Design review of the part built by this model. Coordinates are the model's own, in mm. A direction names the side the tool comes from. Coordinates: 2 decimals unless noted, no trailing zeros. Write each loop counter-clockwise with the first axis right and the second up, starting at its lowest first coordinate (ties: lowest second). Pieces come first, ordered by that corner, then holes. Notation, with made-up numbers: (-39.5, 15.25) - (-33.5, 15.25) arc R10 cw to (-33.5, 19.25) - close; hole circle Ø7 at (50.5, 17.5). An arc over 180 degrees is marked (long way). Answer as a JSON object with one key per item and string values.
```python
from build123d import *

# Parameters (mm, degrees)
F0_W     = 38.1
F0_H     = 33.02
F1_DEPTH = 25.4
F2_W     = 38.1
F2_H     = 21.844
F3_DEPTH = 19.05
F4_W     = 5.08
F4_H     = 5.08
F5_DEPTH = 7.62
F6_R     = 5.08


with BuildPart() as f1:
    # F0 (on Front) → F1 (new body)
    with BuildSketch(Plane.XZ):
        with Locations((19.05, 16.51)):
            Rectangle(F0_W, F0_H)
    extrude(amount=F1_DEPTH)

    # F2 (on face) → F3 (cut)
    with BuildSketch(Plane.XZ.offset(25.4)):
        with Locations((19.05, 22.098)):
            Rectangle(F2_W, F2_H)
    extrude(amount=-F3_DEPTH, mode=Mode.SUBTRACT)

    # F4 (on face) → F5 (cut)
    with BuildSketch(Plane.XY.offset(11.176)):
        with Locations((8.89, -15.113)):
            Rectangle(F4_W, F4_H)
        with Locations((29.21, -15.113)):
            Rectangle(F4_W, F4_H)
    extrude(amount=-F5_DEPTH, mode=Mode.SUBTRACT)

    # F6
    f6_edges = [f1.edges().sort_by_distance(p)[0] for p in [
        (19.05, 0, 33.02),
    ]]
    fillet(f6_edges, radius=F6_R)


solid = f1.part
```
(1) Take a section at A-A, the plane z = 6.5. Write out the cut boundary in (x, y).
Solved:
{"outline": "(0, -25.4) - (38.1, -25.4) - (38.1, 0) - (0, 0) - close; hole (6.35, -17.65) - (11.43, -17.65) - (11.43, -12.57) - (6.35, -12.57) - close; hole (26.67, -17.65) - (31.75, -17.65) - (31.75, -12.57) - (26.67, -12.57) - close"}
(2) Tool access review of faces 4 (the face through (19, -6, 33.02)), 5 (the face through (19, -16, 11.176)), 6 (the face through (9, -15, 3.556)): name each direction out of +Z, -Z, +X, -X, +Y, -Y from which nothing blocks a thin tool from reaching the whole face with its end or side.
Solved:
{"face 4": "+Z, +X, -X, +Y, -Y", "face 5": "+Z, +X, -X, -Y", "face 6": "+Z"}
(3) The part is to be moulded in two halves that separate along X. For faces 1 (the face through (19, -25.4, 6)), 2 (the face through (6.35, -15, 7)), 3 (the face through (0, -10, 9)), say which applies: pulls with the +X half, pulls with the -X half, needs draft (parallel to the pull), parting line crosses it, or undercut.
Solved:
{"face 1": "needs draft", "face 2": "undercut", "face 3": "pulls with the -X half"}
(4) Take a section at C-C, the plane y = -14.5. Write out the cut boundary in (x, z), and give its area (3 significant figures).
Solved:
{"outline": "(0, 0) - (38.1, 0) - (38.1, 11.18) - (31.75, 11.18) - (31.75, 3.56) - (26.67, 3.56) - (26.67, 11.18) - (11.43, 11.18) - (11.43, 3.56) - (6.35, 3.56) - (6.35, 11.18) - (0, 11.18) - close", "area": "348 mm^2"}
(5) Take a section at D-D, the plane x = 23. Write out the cut boundary in (y, z), and give its area (3 significant figures).
Solved:
{"outline": "(-25.4, 0) - (0, 0) - (0, 27.94) arc R5.08 ccw to (-5.08, 33.02) - (-6.35, 33.02) - (-6.35, 11.18) - (-25.4, 11.18) - close", "area": "417 mm^2"}
(6) For pin 1 (5.5 mm diameter, centred on x = 30, y = -15, fed in from +Z), flat-tipped, find the tip position at first contact; note if it passes through.
Solved:
{"pin 1": "stops at z = 11.18"}
(7) To check wall thickness, follow line 1 (Z direction, x = 12.5, y = -21.5); line 2 (Y direction, x = 6, z = 27.5); line 3 (Z direction, x = 27, y = -16.25). State the ranges of each line that lie inside material, in increasing order. Write a range as from..to.
Solved:
{"line 1": "z = 0..11.18", "line 2": "y = -6.35..0", "line 3": "z = 0..3.56"}
(8) Take a section at B-B, the plane x = 9. Write out the cut boundary in (y, z), and give its area (3 significant figures).
Solved:
{"outline": "(-25.4, 0) - (0, 0) - (0, 27.94) arc R5.08 ccw to (-5.08, 33.02) - (-6.35, 33.02) - (-6.35, 11.18) - (-12.57, 11.18) - (-12.57, 3.56) - (-17.65, 3.56) - (-17.65, 11.18) - (-25.4, 11.18) - close", "area": "378 mm^2"}
